Build history of the part. All positions in model axes, mm. Give positions to 0.01 mm unless a question says otherwise; leave off trailing zeros. Order: outer loops, then holes, each group sorted by start corner. A loop starts at its lowest first (then second) coordinate and runs counter-clockwise, first axis right, second up. Notation, with made-up numbers: (-26, -37) -> (31, -37) arc R28 cw to (31, -15) -> close; hole circle Ø9 at (50, 13). An arc over 180 degrees is marked (long way). One line per question, with ' | ' between items. Start each with the question number.
(1) Drill centre lines: L1, parallel to Y at x = 137.5, z = -0.1; L2, parallel to X at y = -74, z = -0.35; L3, parallel to X at y = -72, z = -1.2. Where is each one in solid material? Low to high. Write a range as from..to.
(2) Cut at A-A (x = 281). Give the cut face in (y, z).
(3) Cut at C-C (y = -31.5). Give the cut face in (x, z), then the cut area to 3 significant figures.
(4) Pin check, flat tips, straight feed: pin 1 Ø1.5 at (x, z) = (212, 0.5) entering from -Y; pin 2 Ø0.9 at (x, z) = (278.5, 0.5) entering from +Y; pin 3 Ø1.5 at (y, z) = (-20.5, 0.5) entering from -X. Stop position of each tip, or through.
(5) Cut at B-B (x = 215). Give the cut face in (y, z), then the cut area to 3 significant figures.
from build123d import *

# Parameters (mm, degrees)
BOSS_EXTRUDE1_DEPTH = 1.5
SKETCH3_W           = 13.3
SKETCH3_H           = 3
CUT_EXTRUDE1_DEPTH  = 10
FILLET1_R           = 1
SKETCH4_W           = 2
SKETCH4_H           = 7.019019915
CUT_EXTRUDE2_DEPTH  = 10
BOSS_EXTRUDE2_DEPTH = 3


with BuildPart() as part:
    # Sketch2 → Boss-Extrude1 (new, symmetric)
    with BuildSketch(Plane.XY):
        with BuildLine():
            Line((299.5, -67.353443934), (293.5, -67.353443934))
            ThreePointArc((293.5, -67.353443934), (292.085786438, -67.939230372), (291.5, -69.353443934))
            Line((291.5, -69.353443934), (291.5, -85.649534053))
            Line((291.5, -85.649534053), (271.5, -85.649534053))
            Line((271.5, -85.649534053), (271.5, -65.603161932))
            ThreePointArc((271.5, -65.603161932), (270.728442335, -62.934777511), (268.651889832, -61.089918071))
            ThreePointArc((268.651889832, -61.089918071), (217.204334173, -39.861711653), (163.781589842, -24.257285386))
            Line((163.781589842, -24.257285386), (141, -24.257285386))
            ThreePointArc((141, -24.257285386), (140.292893219, -23.964392167), (140, -23.257285386))
            Line((140, -23.257285386), (140, -19.257285386))
            Line((140, -19.257285386), (126, -19.257285386))
            ThreePointArc((126, -19.257285386), (125.292893219, -18.964392167), (125, -18.257285386))
            Line((125, -18.257285386), (125, -17.551725847))
            ThreePointArc((125, -17.551725847), (124.759050209, -16.900693759), (124.152314439, -16.563393762))
            ThreePointArc((124.152314439, -16.563393762), (89.724531973, -12.428170907), (55.097618142, -10.598112953))
            ThreePointArc((55.097618142, -10.598112953), (55.000467449, -10.596696958), (54.903307584, -10.596224945))
            Line((54.903307584, -10.596224945), (27, -10.596224945))
            ThreePointArc((27, -10.596224945), (25.585786438, -10.010438507), (25, -8.596224945))
            Line((25, -8.596224945), (25, -5.5))
            ThreePointArc((25, -5.5), (25.585786438, -4.085786438), (27, -3.5))
            Line((27, -3.5), (45, -3.5))
            Line((45, -3.5), (45, -1.500945781))
            ThreePointArc((45, -1.500945781), (45.293562303, -0.793170548), (46.001891561, -0.50094757))
            ThreePointArc((46.001891561, -0.50094757), (176.838494864, -17.170276226), (299.5, -65.649534053))
            Line((299.5, -65.649534053), (299.5, -67.353443934))
        make_face()
    extrude(amount=BOSS_EXTRUDE1_DEPTH, both=True)

    # Sketch3 → Cut-Extrude1 (cut)
    with BuildSketch(Plane.XY.offset(1.5)):
        with Locations((278.15, -71.353443934)):
            Rectangle(SKETCH3_W, SKETCH3_H)
        with Locations((278.15, -79.353443934)):
            Rectangle(SKETCH3_W, SKETCH3_H)
    extrude(amount=-CUT_EXTRUDE1_DEPTH, mode=Mode.SUBTRACT)

    # Fillet1
    fillet1_edges = [part.edges().sort_by_distance(p)[0] for p in [
        (271.5, -72.853443934, 0),
        (271.5, -69.853443934, 0),
        (271.5, -80.853443934, 0),
        (271.5, -77.853443934, 0),
    ]]
    fillet(fillet1_edges, radius=FILLET1_R)

    # Sketch4 → Cut-Extrude2 (cut)
    with BuildSketch(Plane.XY.offset(1.5)):
        with Locations((298.5, -66.105228371)):
            Rectangle(SKETCH4_W, SKETCH4_H)
    extrude(amount=-CUT_EXTRUDE2_DEPTH, mode=Mode.SUBTRACT)

    # Sketch5 → Boss-Extrude2 (add)
    with BuildSketch(Plane.XY.offset(1.5)):
        with BuildLine():
            Line((140, -19.257285386), (140, -22.257285386))
            Line((140, -22.257285386), (127, -22.257285386))
            ThreePointArc((127, -22.257285386), (125.585786438, -22.843071823), (125, -24.257285386))
            Line((125, -24.257285386), (125, -25.257285386))
            ThreePointArc((125, -25.257285386), (125.585786438, -26.671498948), (127, -27.257285386))
            Line((127, -27.257285386), (175.902657485, -27.257285386))
            Line((175.902657485, -27.257285386), (184.756236065, -23.311413726))
            Line((184.756236065, -23.311413726), (140, -19.257285386))
        make_face()
    extrude(amount=-BOSS_EXTRUDE2_DEPTH)


solid = part.part
Result set:
1) L1: y = -27.26..-22.26, -19.26..-8.64 | L2: x = 271.5..291.5 | L3: x = 284.8..291.5
2) outline: (-85.65, -1.5) -> (-80.85, -1.5) -> (-80.85, 1.5) -> (-85.65, 1.5) -> close; (-77.85, -1.5) -> (-72.85, -1.5) -> (-72.85, 1.5) -> (-77.85, 1.5) -> close; (-69.85, -1.5) -> (-55.98, -1.5) -> (-55.98, 1.5) -> (-69.85, 1.5) -> close
3) outline: (191.24, -1.5) -> (223.54, -1.5) -> (223.54, 1.5) -> (191.24, 1.5) -> close | area: 96.9 mm2
4) pin 1: stops at y = -38.32 | pin 2: stops at y = -54.53 | pin 3: stops at x = 140
5) outline: (-39.09, -1.5) -> (-28.52, -1.5) -> (-28.52, 1.5) -> (-39.09, 1.5) -> close | area: 31.7 mm2
